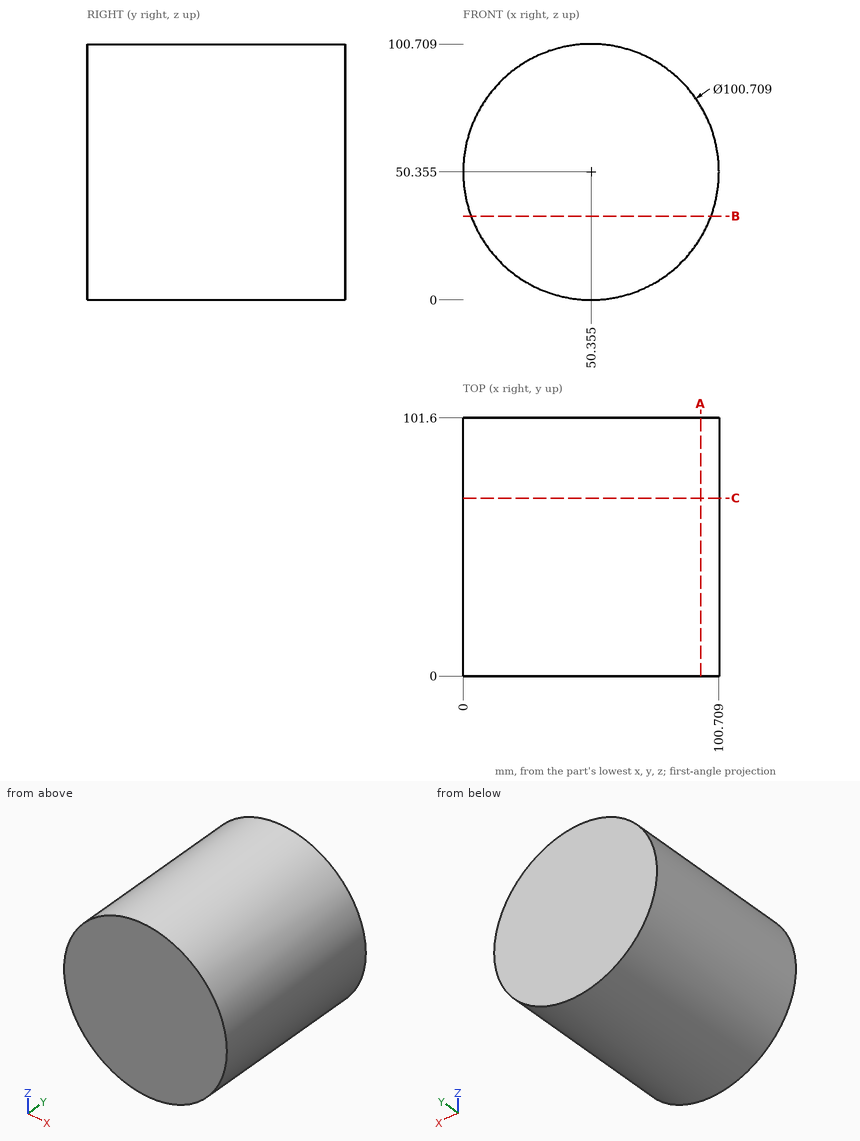
Drawing for the job (mm, zero at the part's lowest x, y, z). Coordinates: 2 decimals unless noted, no trailing zeros. Order: outer loops, then holes, each group sorted by start corner. A loop starts at its lowest first (then second) coordinate and runs counter-clockwise, first axis right, second up. Notation, with made-up numbers: (58.5, 69.5) -> (107.5, 69.5) arc R17 cw to (107.5, 78.5) -> close; hole circle Ø1 at (44.25, 32). An arc over 180 degrees is marked (long way). One line per item, written item: value.
(1) Slice it at C-C, the plane y = 70. List the corners of the cut face in (x, z) (1 decimal).
Checked values:
outline: circle Ø100.7 at (50.4, 50.4)
(2) Slice it at B-B, the plane z = 33. List the corners of the cut face in (x, y) (1 decimal), plus the area to 4 significant figures.
Checked values:
outline: (3.1, 0) -> (97.6, 0) -> (97.6, 101.6) -> (3.1, 101.6) -> close
area: 9,605 mm2
(3) Drop flat-ended pins along their axis: pin 1 Ø3 at (y, z) = (30, 36) entering from -X; pin 2 Ø3 at (y, z) = (79, 44.5) entering from -X; pin 3 Ø6 at (y, z) = (62, 79) entering from -X. Give the stop position or say it passes through.
Checked values:
pin 1: x = 1.67
pin 2: x = 0.19
pin 3: x = 7.02
(4) Probe line 1 (Z direction, x = 49, y = 69); line 2 (X direction, y = 46, z = 19) (1 decimal); line 3 (Z direction, x = 14.5, y = 16). List the from-to ranges inside material, lowest first. Write a range as [from, to].
Checked values:
line 1: [0.02, 100.69]
line 2: [11, 89.8]
line 3: [15, 85.71]
(5) Slice it at A-A, the plane x = 93.5. List the corners of the cut face in (y, z), plus the area to 3 significant figures.
Checked values:
outline: (0, 24.39) -> (101.6, 24.39) -> (101.6, 76.32) -> (0, 76.32) -> close
area: 5,280 mm2
